from build123d import *

# Parameters (mm, degrees)
SKETCH1_R                            = 121.5
SKETCH1_R_2                          = 43.5
BOSS_EXTRUDE1_DEPTH                  = 9.525
CUT_EXTRUDE1_START                   = 9.525
SKETCH1_4_R                          = 52.1208
SKETCH1_4_R_2                        = 47.371
CUT_EXTRUDE1_DEPTH                   = 2.8448
CIRPATTERN1_COUNT                    = 16
SKETCH5_R                            = 6.35
CUBE_5_16_CLEARANCE_THRU_HOLES_DEPTH = 173.090748226
F_5_16_18_TAPPED_HOLE1_D             = 6.5278
CIRPATTERN3_COUNT                    = 8
BOTTOM_ISO160_R                      = 76.5
BOTTOM_ISO160_R_2                    = 70.1548
CUT_EXTRUDE3_DEPTH                   = 2.79
FILLET1_R                            = 0.254


with BuildPart() as part:
    # Sketch1 → Boss-Extrude1 (new body)
    with BuildSketch(Plane(origin=(0, 0, 0), x_dir=(1, 0, 0), z_dir=(0, 1, 0))):
        with Locations(Location((0, 0, 0), (0, 0, 90))):
            Circle(SKETCH1_R)
        with Locations(Location((0, 0, 0), (0, 0, 90))):
            Circle(SKETCH1_R_2, mode=Mode.SUBTRACT)
    extrude(amount=BOSS_EXTRUDE1_DEPTH)

    # Sketch1<4> → Cut-Extrude1 (cut)
    with BuildSketch(Plane(origin=(0, 0, 0), x_dir=(1, 0, 0), z_dir=(0, 1, 0)).offset(CUT_EXTRUDE1_START)):
        with Locations(Location((0, 0, 0), (0, 0, 270))):
            Circle(SKETCH1_4_R)
        with Locations(Location((0, 0, 0), (0, 0, 270))):
            Circle(SKETCH1_4_R_2, mode=Mode.SUBTRACT)
    extrude(amount=-CUT_EXTRUDE1_DEPTH, mode=Mode.SUBTRACT)

    # Sketch4 → M5x0.8 Tapped Hole2 (revolve, cut)
    with BuildSketch(Plane(origin=(60, 9.525, 0), x_dir=(0, 0, 1), z_dir=(1, 0, 0))):
        Polygon((0, 0), (0, 7), (2.1, 5.7381927), (2.1, 0), align=None)
    m5x0_8_tapped_hole2 = revolve(axis=Axis((60, 15.875, 0), (0, -1, 0)), mode=Mode.SUBTRACT)

    # CirPattern1: M5x0.8 Tapped Hole2 ×16 about axis, 12 skipped
    cirpattern1_axis = Axis((0, 9.525, 0), (0, -1, 0))
    add([m5x0_8_tapped_hole2.rotate(cirpattern1_axis, i * 360 / CIRPATTERN1_COUNT) for i in range(1, CIRPATTERN1_COUNT) if i not in (1, 2, 3, 4, 5, 7, 9, 10, 11, 12, 13, 15)], mode=Mode.SUBTRACT)

    # Sketch5 → Cube_5/16_Clearance_Thru Holes (cut, through all)
    with BuildSketch(Plane(origin=(0, 0, 0), x_dir=(1, 0, 0), z_dir=(0, 1, 0))):
        with Locations(Location((11.289074033, -107.4083647, 0), (0, 0, 270))):
            Circle(SKETCH5_R)
        with Locations(Location((47.344083853, -97.069757, 0), (0, 0, 270))):
            Circle(SKETCH5_R)
        with Locations(Location((-67.966602233, -83.931763837, 0), (0, 0, 270))):
            Circle(SKETCH5_R)
        with Locations(Location((-35.161360681, -102.116006165, 0), (0, 0, 270))):
            Circle(SKETCH5_R)
        with Locations(Location((-107.4083647, -11.289074033, 0), (0, 0, 270))):
            Circle(SKETCH5_R)
        with Locations(Location((-97.069757, -47.344083853, 0), (0, 0, 270))):
            Circle(SKETCH5_R)
        with Locations(Location((-83.931763837, 67.966602233, 0), (0, 0, 270))):
            Circle(SKETCH5_R)
        with Locations(Location((-102.116006165, 35.161360681, 0), (0, 0, 270))):
            Circle(SKETCH5_R)
        with Locations(Location((-11.289074033, 107.4083647, 0), (0, 0, 270))):
            Circle(SKETCH5_R)
        with Locations(Location((-47.344083853, 97.069757, 0), (0, 0, 270))):
            Circle(SKETCH5_R)
        with Locations(Location((67.966602233, 83.931763837, 0), (0, 0, 270))):
            Circle(SKETCH5_R)
        with Locations(Location((35.161360681, 102.116006165, 0), (0, 0, 270))):
            Circle(SKETCH5_R)
        with Locations(Location((107.4083647, 11.289074033, 0), (0, 0, 270))):
            Circle(SKETCH5_R)
        with Locations(Location((97.069757, 47.344083853, 0), (0, 0, 270))):
            Circle(SKETCH5_R)
        with Locations(Location((83.931763837, -67.966602233, 0), (0, 0, 270))):
            Circle(SKETCH5_R)
        with Locations(Location((102.116006165, -35.161360681, 0), (0, 0, 270))):
            Circle(SKETCH5_R)
    extrude(amount=CUBE_5_16_CLEARANCE_THRU_HOLES_DEPTH, mode=Mode.SUBTRACT)

    # 5/16-18 Tapped Hole1 (through all)
    with Locations(Plane(origin=(-62.251463664, 0, -78.260815685), x_dir=(0, 0, -1), z_dir=(0, -1, 0))):
        with Locations((0, 0)):
            f_5_16_18_tapped_hole1 = Hole(F_5_16_18_TAPPED_HOLE1_D / 2)

    # CirPattern3: 5/16-18 Tapped Hole1 ×8 about axis
    cirpattern3_axis = Axis((0, 0, 0), (0, 1, 0))
    for i in range(1, CIRPATTERN3_COUNT):
        add(f_5_16_18_tapped_hole1.rotate(cirpattern3_axis, i * 360 / CIRPATTERN3_COUNT), mode=Mode.SUBTRACT)

    # Bottom_Iso160 → Cut-Extrude3 (cut)
    with BuildSketch(Plane(origin=(0, 0, 0), x_dir=(1, 0, 0), z_dir=(0, 1, 0))):
        with Locations(Location((0, 0, 0), (0, 0, 270))):
            Circle(BOTTOM_ISO160_R)
        with Locations(Location((0, 0, 0), (0, 0, 270))):
            Circle(BOTTOM_ISO160_R_2, mode=Mode.SUBTRACT)
    extrude(amount=CUT_EXTRUDE3_DEPTH, mode=Mode.SUBTRACT)

    # Fillet1
    fillet1_edges = [part.edges().sort_by_distance(p)[0] for p in [
        (0, 6.6802, -52.1208),
        (0, 6.6802, -47.371),
    ]]
    fillet(fillet1_edges, radius=FILLET1_R)


solid = part.part
Could you check a few things on this model? Use its own coordinates, in mm. A direction names the side the tool comes from. Round coordinates to 2 decimals unless told otherwise and drop trailing zeros.
(1) Imagine slicing it at A-A (y = 5.25). Count the separate pieces of the cut face and the enclosed holes in it, plus the area to 3 significant figures.
Response values:
separate pieces: 1
enclosed holes: 29
area: 38,100 mm2
(2) I'm going to push flat-ended pins straight in: pin 1 (1 mm diameter, centred on x = 54, y = 2.5, fed in from -Z); pin 2 (6 mm diameter, centred on x = 78.26, z = -62.25, fed in from -Y); pin 3 (2 mm diameter, centred on x = 46.5, y = 8, fed in from +Z); pin 4 (4 mm diameter, centred on y = 2, z = 21.5, fed in from +X) (3 decimals). Where does each tip first touch, or does it pass through?
Response values:
pin 1: stops at z = -109.09
pin 2: passes through
pin 3: stops at z = 112.66
pin 4: stops at x = 119.925
(3) Which directions (+Z, -Z, +X, -X, +Y, -Y) give clear straight access to the entire face, cutting with the end or side of a thin tool? Please do faces 1 (the cylindrical face through (21.073, 1.375, 66.915)), 2 (the cylindrical face through (96.48, 4.7, 38.09)), 3 (the flat face through (-42, 6.68, 23)).
Response values:
face 1: -Y
face 2: +Y, -Y
face 3: +Y
(4) If we mould it in two halves opening along Z, with no side actions, what happens to faces 4 (the flat face through (38.4, 9.525, -20.8)), 5 (the cylindrical face through (96.17, 4.83, 12.03))? For each: released by +Z, released by -Z, zero draft, split by the parting line, or undercut.
Response values:
face 4: zero draft
face 5: undercut
(5) Please list where these lines run through material, in increasing order: line 1 along X through (y, z) = (2.5, -1); line 2 along X through (y, z) = (6.9, 0); line 3 along X through (y, z) = (7.75, -3).
Response values:
line 1: x = -121.5 to -76.49, -70.15 to -43.49, 43.49 to 70.15, 76.49 to 121.5
line 2: x = -121.5 to -62.1, -57.9 to -52.12, -47.37 to -43.5, 43.5 to 47.37, 52.12 to 57.9, 62.1 to 121.5
line 3: x = -121.46 to -52.03, -47.28 to -43.4, 43.4 to 47.28, 52.03 to 121.46
